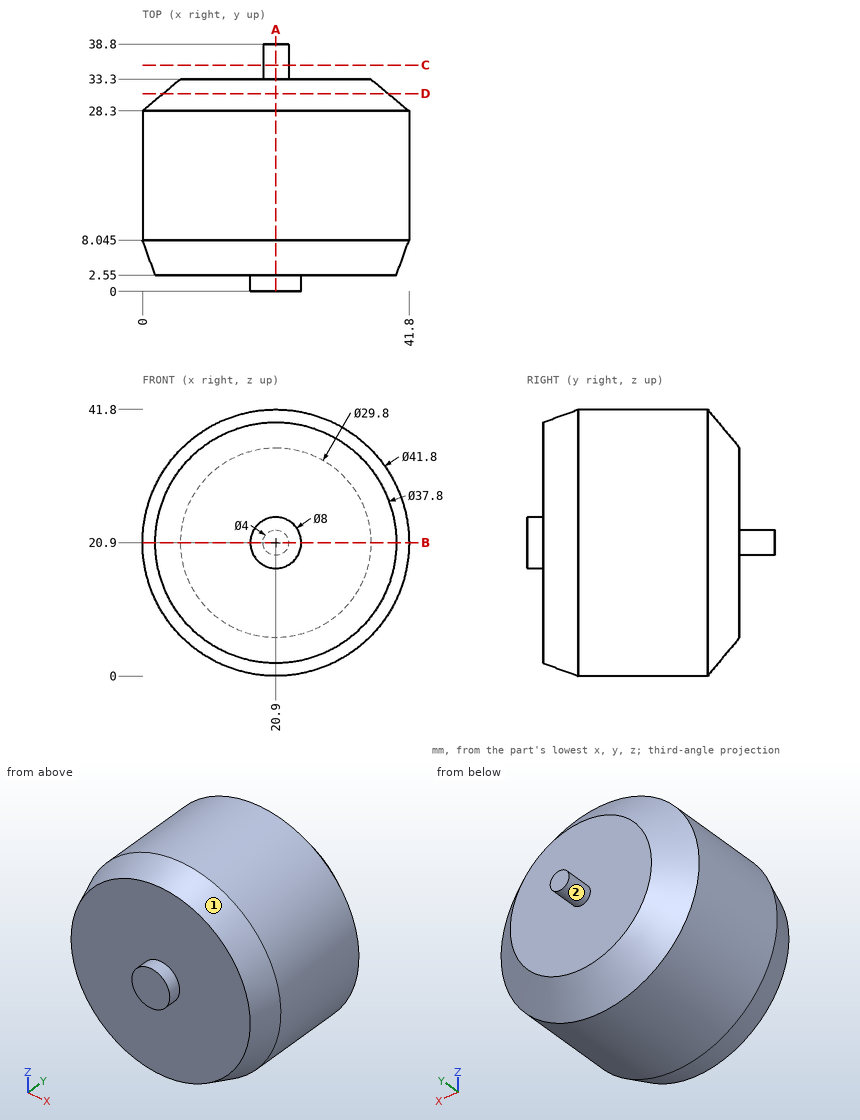
Job drawing, mm, ordinate dimensions from the low corner. One solid piece. A direction names the side the tool comes from. Round coordinates to 2 decimals unless told otherwise and drop trailing zeros. Order: outer loops, then holes, each group sorted by start corner. A loop starts at its lowest first (then second) coordinate and runs counter-clockwise, first axis right, second up. Notation, with made-up numbers: (-19, 73.25) -> (33, 73.25) arc R20 ccw to (33, 93.25) -> close; hole circle Ø2 at (62.25, 77.25). An arc over 180 degrees is marked (long way). Answer in a Markdown table with one row per item.
1) Band-saw the part on B-B on z = 20.9. Give the cut face in (x, y) (3 decimals).
Values:
| item | result |
|---|---|
| outline | (0, 8.045) -> (2, 2.55) -> (16.9, 2.55) -> (16.9, 0) -> (24.9, 0) -> (24.9, 2.55) -> (39.8, 2.55) -> (41.8, 8.045) -> (41.8, 28.3) -> (35.8, 33.3) -> (22.9, 33.3) -> (22.9, 38.8) -> (18.9, 38.8) -> (18.9, 33.3) -> (6, 33.3) -> (0, 28.3) -> close |
2) Band-saw the part on A-A on x = 20.9. Give the cut face in (y, z) (3 decimals), and give its area (3 significant figures).
Values:
| item | result |
|---|---|
| outline | (0, 16.9) -> (2.55, 16.9) -> (2.55, 2) -> (8.045, 0) -> (28.3, 0) -> (33.3, 6) -> (33.3, 18.9) -> (38.8, 18.9) -> (38.8, 22.9) -> (33.3, 22.9) -> (33.3, 35.8) -> (28.3, 41.8) -> (8.045, 41.8) -> (2.55, 39.8) -> (2.55, 24.9) -> (0, 24.9) -> close |
| area | 1,290 mm2 |
3) Which spindle directions (+Z, -Z, +X, -X, +Y, -Y) get a long thin tool onto all of the face, cutting with end or side? Do the marked faces 1 and 2. Say none if no direction does.
Values:
| item | result |
|---|---|
| face 1 | -Y |
| face 2 | +Y |
4) Wall check: L1, parallel to X at y = 18.5, z = 21.5; L2, parallel to Y at x = 10, z = 30.5; L3, parallel to Y at x = 31.5, z = 4. Give the ranges that are in metal, low to high.
Values:
| item | result |
|---|---|
| L1 | 0.01 to 41.79 |
| L2 | 2.55 to 33.3 |
| L3 | 5.43 to 29.09 |
5) Pin check, flat tips, straight feed: P1, Ø1.5, axis at y = 5.5, z = 25, coming from the -X side; P2, Ø5, axis at x = 13, z = 27, coming from the -Y side; P3, Ø8, axis at x = 34.5, z = 16, coming from the +Y side; P4, Ø15, axis at x = 23, z = 22, coming from the +Y side. Stop position of each tip, or through.
Values:
| item | result |
|---|---|
| P1 | x = 1.04 |
| P2 | y = 2.55 |
| P3 | y = 33.3 |
| P4 | y = 38.8 |
6) Band-saw the part on D-D on y = 31. Give the cut face in (x, z).
Values:
| item | result |
|---|---|
| outline | circle Ø35.32 at (20.9, 20.9) |
7) Band-saw the part on C-C on y = 35.5. Give the cut face in (x, z).
Values:
| item | result |
|---|---|
| outline | circle Ø4 at (20.9, 20.9) |
